Part print with two shaded views. Sizes in mm from the minimum x, y, z corner. Coordinates: 2 decimals unless noted, no trailing zeros. Loops run counter-clockwise (first coordinate to the right, second up) from the corner with the lowest first, then second, coordinate; pieces in that order, holes last. Notation, with made-up numbers: (51.25, 55) -> (103.25, 55) arc R18 ccw to (103.25, 83) -> close; hole circle Ø11 at (80.5, 62). An arc over 180 degrees is marked (long way). Use one line per item in the form item = value.
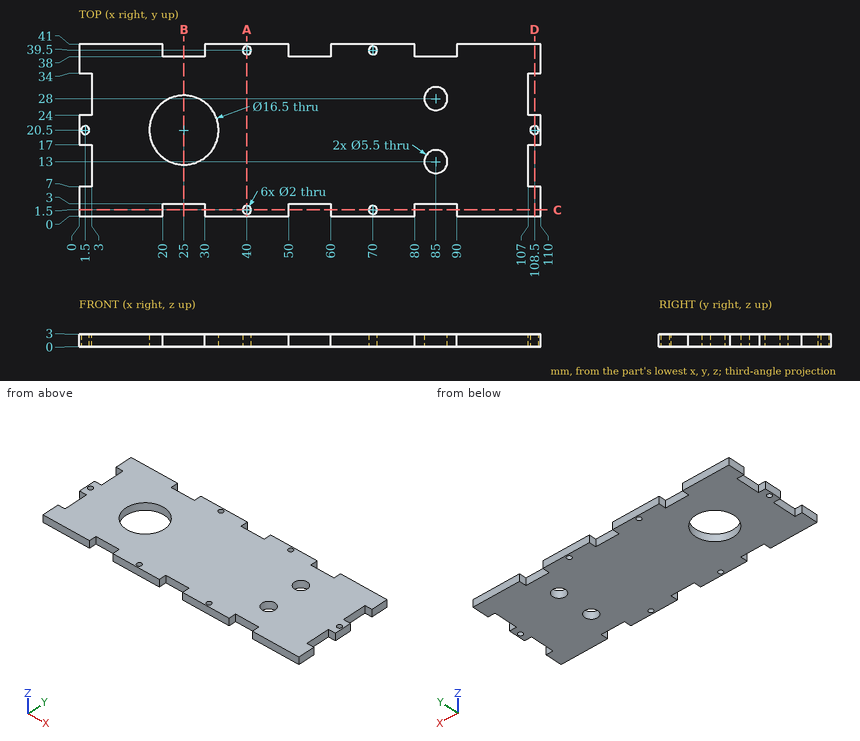
Q1. Band-saw the part on C-C, the plane y = 1.5. Write the cut outline in (x, z), and give its area (3 significant figures).
Result:
outline = (0, 0) -> (20, 0) -> (20, 3) -> (0, 3) -> close; (30, 0) -> (39, 0) -> (39, 3) -> (30, 3) -> close; (41, 0) -> (50, 0) -> (50, 3) -> (41, 3) -> close; (60, 0) -> (69, 0) -> (69, 3) -> (60, 3) -> close; (71, 0) -> (80, 0) -> (80, 3) -> (71, 3) -> close; (90, 0) -> (110, 0) -> (110, 3) -> (90, 3) -> close
area = 228 mm2
Q2. Band-saw the part on B-B, the plane x = 25. Write the cut outline in (y, z), and give its area (3 significant figures).
Result:
outline = (3, 0) -> (12.25, 0) -> (12.25, 3) -> (3, 3) -> close; (28.75, 0) -> (38, 0) -> (38, 3) -> (28.75, 3) -> close
area = 55.5 mm2
Q3. Band-saw the part on A-A, the plane x = 40. Write the cut outline in (y, z), and give its area (3 significant figures).
Result:
outline = (0, 0) -> (0.5, 0) -> (0.5, 3) -> (0, 3) -> close; (2.5, 0) -> (38.5, 0) -> (38.5, 3) -> (2.5, 3) -> close; (40.5, 0) -> (41, 0) -> (41, 3) -> (40.5, 3) -> close
area = 111 mm2
Q4. Wall check: line 1 along Y through (x, z) = (70, 1.05); line 2 along Y through (x, z) = (84.5, 2.85); line 3 along Y through (x, z) = (25, 0.65). Give the ranges that are in metal, low to high.
Result:
line_1 = 0 to 0.5, 2.5 to 38.5, 40.5 to 41
line_2 = 3 to 10.3, 15.7 to 25.3, 30.7 to 38
line_3 = 3 to 12.25, 28.75 to 38
Q5. Band-saw the part on D-D, the plane x = 108.5. Write the cut outline in (y, z).
Result:
outline = (0, 0) -> (7, 0) -> (7, 3) -> (0, 3) -> close; (17, 0) -> (19.5, 0) -> (19.5, 3) -> (17, 3) -> close; (21.5, 0) -> (24, 0) -> (24, 3) -> (21.5, 3) -> close; (34, 0) -> (41, 0) -> (41, 3) -> (34, 3) -> close
Q6. Pin check, flat tips, straight feed: pin 1 Ø1.5 at (x, z) = (55.5, 1.5) entering from -Y; pin 2 Ø0.9 at (y, z) = (27, 1.5) entering from -X. Stop position of each tip, or through.
Result:
pin_1 = 3
pin_2 = 3
